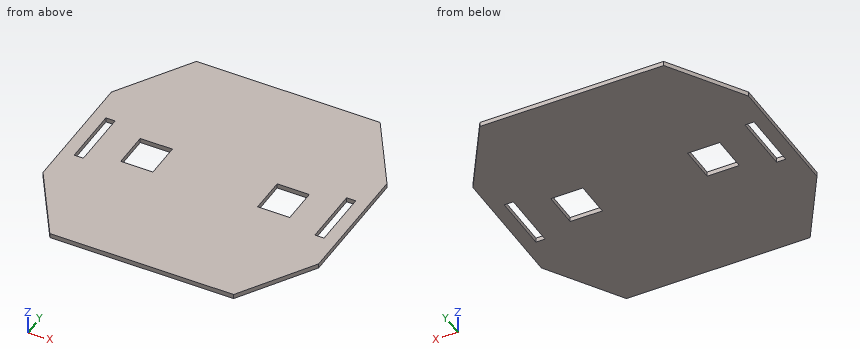
from build123d import *

# Parameters (mm, degrees)
BOSS_EXTRU_1_DEPTH      = 5
ESQUISSE5_W             = 35
ESQUISSE5_H             = 40
ESQUISSE5_W_2           = 10
ESQUISSE5_H_2           = 65
ENL_V_MAT_EXTRU_1_DEPTH = 20


with BuildPart() as part:
    # Esquisse3 → Boss.-Extru.1 (new body)
    with BuildSketch(Plane.XY):
        Polygon((-100, 150), (-150, 70), (-150, -70), (-100, -150), (100, -150), (150, -70), (150, 70), (100, 150), align=None)
    extrude(amount=BOSS_EXTRU_1_DEPTH)

    # Esquisse5 → Enlèv. mat.-Extru.1 (cut)
    with BuildSketch(Plane.XY.offset(5)):
        with Locations((-74.5, 0)):
            Rectangle(ESQUISSE5_W, ESQUISSE5_H)
        with Locations((74.5, 0)):
            Rectangle(ESQUISSE5_W, ESQUISSE5_H)
        with Locations((-130.993475803, 0)):
            Rectangle(ESQUISSE5_W_2, ESQUISSE5_H_2)
        with Locations((130.993475803, 0)):
            Rectangle(ESQUISSE5_W_2, ESQUISSE5_H_2)
    extrude(amount=-ENL_V_MAT_EXTRU_1_DEPTH, mode=Mode.SUBTRACT)


solid = part.part
Input: part model. Units: mm. Frame: model coordinates. Coordinates: 2 decimals unless noted, no trailing zeros. Loops run counter-clockwise (first coordinate to the right, second up) from the corner with the lowest first, then second, coordinate; pieces in that order, holes last. Notation, with made-up numbers: (22.25, -23.5) -> (38.25, -23.5) arc R18 ccw to (38.25, -4.5) -> close; hole circle Ø4 at (10.25, -26.75). An arc over 180 degrees is marked (long way). Write item = value, one per line. Start each with the question number.
Item 1: Cut plane B-B, the plane y = 14. Return loops of the section in (x, z).
Item 2: Cut plane A-A, the plane x = 85.5. Return loops of the section in (y, z), plus the area to 3 significant figures.
Item 3: First-contact query: P1, Ø5, axis at x = 85.5, y = -38, coming from the -Z side; P2, Ø1.5, axis at x = 129, z = 3.5, coming from the +Y side. Flat tips, straight axial feed; report the tip coordinate or a pass-through.
Item 4: Cut plane C-C, the plane z = 3.9. Return loops of the section in (x, y).
Item 5: Material intervals for line 1 (X direction, y = -4, z = 2.95); line 2 (X direction, y = -26.5, z = 2.6); line 3 (Y direction, x = -57.5, z = 3.2), sorted ascending.
Item 6: Cut plane D-D, the plane x = -116. Return loops of the section in (y, z).
Ans:
q1.outline = (-150, 0) -> (-135.99, 0) -> (-135.99, 5) -> (-150, 5) -> close; (-125.99, 0) -> (-92, 0) -> (-92, 5) -> (-125.99, 5) -> close; (-57, 0) -> (57, 0) -> (57, 5) -> (-57, 5) -> close; (92, 0) -> (125.99, 0) -> (125.99, 5) -> (92, 5) -> close; (135.99, 0) -> (150, 0) -> (150, 5) -> (135.99, 5) -> close
q2.outline = (-150, 0) -> (-20, 0) -> (-20, 5) -> (-150, 5) -> close; (20, 0) -> (150, 0) -> (150, 5) -> (20, 5) -> close
q2.area = 1,300 mm²
q3.P1 = 0
q3.P2 = 104.8
q4.outline = (-150, -70) -> (-100, -150) -> (100, -150) -> (150, -70) -> (150, 70) -> (100, 150) -> (-100, 150) -> (-150, 70) -> close; hole (-135.99, -32.5) -> (-125.99, -32.5) -> (-125.99, 32.5) -> (-135.99, 32.5) -> close; hole (-92, -20) -> (-57, -20) -> (-57, 20) -> (-92, 20) -> close; hole (57, -20) -> (92, -20) -> (92, 20) -> (57, 20) -> close; hole (125.99, -32.5) -> (135.99, -32.5) -> (135.99, 32.5) -> (125.99, 32.5) -> close
q5.line_1 = -150 to -135.99, -125.99 to -92, -57 to 57, 92 to 125.99, 135.99 to 150
q5.line_2 = -150 to -135.99, -125.99 to 125.99, 135.99 to 150
q5.line_3 = -150 to -20, 20 to 150
q6.outline = (-124.4, 0) -> (124.4, 0) -> (124.4, 5) -> (-124.4, 5) -> close
